The listing builds one solid part. Answer for the finished solid, in the listing's coordinates (mm). A direction names the side the tool comes from. Coordinates: 2 decimals unless noted, no trailing zeros. Loops run counter-clockwise (first coordinate to the right, second up) from the corner with the lowest first, then second, coordinate; pieces in that order, holes last. Notation, with made-up numbers: (4.25, -6) - (10.25, -6) arc R26 ccw to (10.25, 20) - close; hole circle Ø11 at (-35.75, 53). An arc over 180 degrees is marked (long way). Write each question's results on one line, items separated by ' | '. Start each with the question number.
(1) For faces 5 (the flat face through (-9.5, 43, 0)), 6 (the flat face through (11, 18, 0)), 7 (the cylindrical face through (-10.6, 42.37, 32.64)), determine the directions among +Z, -Z, +X, -X, +Y, -Y from which every point of the face is accessible in a straight line to the end or side of a thin tool.
(2) Find section A-A on y = 77. Determine the outline of the cut face in (x, z), then the cut area to 3 significant figures.
(3) Find section B-B on x = -3. Determine the outline of the cut face in (y, z), then the cut area to 3 significant figures.
(4) Determine the mould class of faces 1 (the flat face through (-11.5, 42, 0)), 2 (the flat face through (11, 19, 2.5)), 3 (the flat face through (0, 0, 0)), 4 (the flat face through (11.5, 42, 0)) for opening direction X: released by +X, released by -X, zero draft, split by the parting line, or undercut.
(5) Find section D-D on z = 14. Determine the outline of the cut face in (x, y), then the cut area to 3 significant figures.
(6) Find section C-C on y = 40.5. Determine the outline of the cut face in (x, z).
(7) Given pin 1 Ø0.6 at (y, z) = (18.5, 0) entering from +X; pin 2 Ø4 at (x, z) = (3, -11.5) entering from +Y; pin 3 Ø1 at (x, y) = (10.5, 18.5) entering from -Z, each flat-ended and moving along its own axis, determine where each tip first touches the part or whether it passes through.
(8) Consider line 1 (Y direction, x = 10, z = 24); line 2 (Y direction, x = 10.2, z = -9); line 3 (X direction, y = 69.5, z = -22.5). Determine where each line is inside the solid, lowest interval first. Write a range as from..to.
Solid Edge part; units mm, degrees
sketch "Sketch1" plane through (0, 0, 0) normal (0, -1, 0) x (1, 0, 0)
  arc A0 (11.5, 30.5) -> (8.5, 33.5) centre (8.5, 30.5) ccw
  line L0 (8.5, 33.5) -> (-8.5, 33.5)
  arc A1 (-8.5, 33.5) -> (-11.5, 30.5) centre (-8.5, 30.5) ccw
  line L1 (-11.5, 30.5) -> (-11.5, -30.5)
  arc A2 (-8.5, -33.5) -> (-11.5, -30.5) centre (-8.5, -30.5) cw
  line L2 (-8.5, -33.5) -> (8.5, -33.5)
  arc A3 (8.5, -33.5) -> (11.5, -30.5) centre (8.5, -30.5) ccw
  line L3 (11.5, -30.5) -> (11.5, 30.5)
  line L4 (-9.5, -30.5) -> (-9.5, 30.5)
  arc A4 (-9.5, 30.5) -> (-8.5, 31.5) centre (-8.5, 30.5) cw
  line L5 (-8.5, 31.5) -> (8.5, 31.5)
  arc A5 (9.5, 30.5) -> (8.5, 31.5) centre (8.5, 30.5) ccw
  line L6 (9.5, 30.5) -> (9.5, -30.5)
  arc A6 (8.5, -31.5) -> (9.5, -30.5) centre (8.5, -30.5) ccw
  line L7 (8.5, -31.5) -> (-8.5, -31.5)
  arc A7 (-8.5, -31.5) -> (-9.5, -30.5) centre (-8.5, -30.5) cw
extrude "Protrusion1" add sketch "Sketch1" against normal blind 88
sketch "Sketch2" plane through (0, 0, 0) normal (0, -1, 0) x (1, 0, 0)
  line L0 (11.5, -30.5) -> (11.5, 30.5)
  arc A0 (11.5, 30.5) -> (8.5, 33.5) centre (8.5, 30.5) ccw
  line L1 (8.5, 33.5) -> (-8.5, 33.5)
  arc A1 (-8.5, 33.5) -> (-11.5, 30.5) centre (-8.5, 30.5) ccw
  line L2 (-11.5, 30.5) -> (-11.5, -30.5)
  arc A2 (-8.5, -33.5) -> (-11.5, -30.5) centre (-8.5, -30.5) cw
  line L3 (-8.5, -33.5) -> (8.5, -33.5)
  arc A3 (8.5, -33.5) -> (11.5, -30.5) centre (8.5, -30.5) ccw
extrude "Boden" add sketch "Sketch2" along normal blind 2
hole "Hole1" at (11.5, 9, -24) direction (-1, 0, 0) diameter 1.5 end up to next
hole "Hole2" at (11.5, 2, 24) direction (-1, 0, 0) diameter 1.5 end up to next
sketch "Sketch3" plane through (11.5, 57, 0) normal (1, 0, 0) x (0, 0, -1)
  line L0 (-2.5, -37) -> (2.5, -37)
  line L1 (2.5, -37) -> (2.5, -39)
  line L2 (2.5, -39) -> (-2.5, -39)
  line L3 (-2.5, -39) -> (-2.5, -37)
  line L4 (-2.5, -47) -> (2.5, -47)
  line L5 (2.5, -47) -> (2.5, -49)
  line L6 (2.5, -49) -> (-2.5, -49)
  line L7 (-2.5, -49) -> (-2.5, -47)
  dimension "D1" = 2.5
  dimension "D2" = 2.5
  dimension "D3" = 2.5
  dimension "D4" = 2.5
extrude "Höhenauschnitt" cut sketch "Sketch3" against normal blind 22
hole "Hole3" at (11.5, 33, -9) direction (-1, 0, 0) diameter 1.5 end up to next
hole "Hole4" at (11.5, 84, -24) direction (-1, 0, 0) diameter 1.5 end up to next
hole "Hole5" at (11.5, 85, 24) direction (-1, 0, 0) diameter 1.5 end up to next
sketch "Sketch4" plane through (11.5, 42.5, 0) normal (1, 0, 0) x (0, 0, -1)
  line L0 (-21, 3.5) -> (-17, 3.5)
  line L1 (-17, 3.5) -> (-17, -11.5)
  line L2 (-17, -11.5) -> (-21, -11.5)
  line L3 (-21, -11.5) -> (-21, 3.5)
  dimension "D1" = 21
  dimension "D2" = 17
extrude "Stromkabelloch" cut sketch "Sketch4" against normal blind 3
Values:
1) face 5: +Y | face 6: +X | face 7: +Z, -X, +Y, -Y
2) outline: (-11.5, -30.5) arc R3 ccw to (-8.5, -33.5) - (8.5, -33.5) arc R3 ccw to (11.5, -30.5) - (11.5, 30.5) arc R3 ccw to (8.5, 33.5) - (-8.5, 33.5) arc R3 ccw to (-11.5, 30.5) - close; hole (-9.5, -30.5) arc R1 ccw to (-8.5, -31.5) - (8.5, -31.5) arc R1 ccw to (9.5, -30.5) - (9.5, 30.5) arc R1 ccw to (8.5, 31.5) - (-8.5, 31.5) arc R1 ccw to (-9.5, 30.5) - close | area: 337 mm²
3) outline: (-2, -33.5) - (88, -33.5) - (88, -31.5) - (0, -31.5) - (0, 31.5) - (88, 31.5) - (88, 33.5) - (-2, 33.5) - close | area: 486 mm²
4) face 1: released by -X | face 2: zero draft | face 3: undercut | face 4: released by +X
5) outline: (-11.5, -2) - (11.5, -2) - (11.5, 88) - (9.5, 88) - (9.5, 0) - (-9.5, 0) - (-9.5, 88) - (-11.5, 88) - close | area: 398 mm²
6) outline: (-11.5, -30.5) arc R3 ccw to (-8.5, -33.5) - (8.5, -33.5) arc R3 ccw to (11.5, -30.5) - (11.5, 17) - (9.5, 17) - (9.5, -30.5) arc R1 cw to (8.5, -31.5) - (-8.5, -31.5) arc R1 cw to (-9.5, -30.5) - (-9.5, 30.5) arc R1 cw to (-8.5, 31.5) - (8.5, 31.5) arc R1 cw to (9.5, 30.5) - (9.5, 21) - (11.5, 21) - (11.5, 30.5) arc R3 ccw to (8.5, 33.5) - (-8.5, 33.5) arc R3 ccw to (-11.5, 30.5) - close
7) pin 1: stops at x = -10.5 | pin 2: stops at y = 0 | pin 3: stops at z = -33.1
8) line 1: y = -2..1.25, 2.75..84.25, 85.75..88 | line 2: y = -2..32.25, 33.75..88 | line 3: x = -11.5..-9.5, 9.5..11.5
